Build history of the part. All positions in model axes, mm. A direction names the side the tool comes from. Give positions to 0.01 mm unless a question says otherwise; leave off trailing zeros. Order: outer loops, then holes, each group sorted by start corner. A loop starts at its lowest first (then second) coordinate and runs counter-clockwise, first axis right, second up. Notation, with made-up numbers: (25, 48.25) - (48, 48.25) arc R15 cw to (48, 54.25) - close; hole circle Ø1 at (-9, 4.5). An arc over 180 degrees is marked (long way). Use a Markdown table: item, result.
from build123d import *

# Parameters (mm, degrees)
ESQUISSE1_W             = 80
ESQUISSE1_H             = 80
BOSS_EXTRU_1_DEPTH      = 7
CONG_1_R                = 8
CONG_2_R                = 2
ESQUISSE2_W             = 75
ESQUISSE2_H             = 75
ENL_V_MAT_EXTRU_1_DEPTH = 4
ENL_V_MAT_EXTRU_2_DEPTH = 2
ENL_V_MAT_EXTRU_3_DEPTH = 2
ESQUISSE6_R             = 0.5
ENL_V_MAT_EXTRU_4_DEPTH = 58
CONG_3_R                = 3


with BuildPart() as part:
    # Esquisse1 → Boss.-Extru.1 (new body)
    with BuildSketch(Plane.XY):
        Rectangle(ESQUISSE1_W, ESQUISSE1_H)
    extrude(amount=BOSS_EXTRU_1_DEPTH)

    # Congé1
    cong_1_edges = [part.edges().sort_by_distance(p)[0] for p in [
        (40, -40, 3.5),
        (-40, -40, 3.5),
        (-40, 40, 3.5),
        (40, 40, 3.5),
    ]]
    fillet(cong_1_edges, radius=CONG_1_R)

    # Congé2
    cong_2_edges = [part.edges().sort_by_distance(p)[0] for p in [
        (0, -40, 7),
        (-40, 0, 7),
        (40, 0, 7),
        (0, 40, 7),
        (37.656854249, 37.656854249, 7),
        (37.656854249, -37.656854249, 7),
        (-37.656854249, 37.656854249, 7),
        (-37.656854249, -37.656854249, 7),
    ]]
    fillet(cong_2_edges, radius=CONG_2_R)

    # Esquisse2 → Enlèv. mat.-Extru.1 (cut)
    with BuildSketch(Plane(origin=(0, 0, 0), x_dir=(-1, 0, 0), z_dir=(0, 0, -1))):
        Rectangle(ESQUISSE2_W, ESQUISSE2_H)
    extrude(amount=-ENL_V_MAT_EXTRU_1_DEPTH, mode=Mode.SUBTRACT)

    # Esquisse3 → Enlèv. mat.-Extru.2 (cut)
    with BuildSketch(Plane.XY.offset(7)):
        Polygon((-38, 0), (-23.013072884, 0), (-20.39099813, 2.622074754), (-16.095973356, -8.657779106), (-14.491160811, -12.872434885), (-8.308759443, 7.774506113), (-6.706462268, -5.579927642), (3.046694847, 2.110487656), (8.341678265, 0), (38, 0), (38, 1.552153758), (8.49875294, 1.552153758), (2.797806202, 3.824451283), (-5.535661698, -2.746531659), (-7.678112046, 15.109838358), (-14.491160811, -7.643232416), (-19.53394935, 5.600443877), (-23.634393227, 1.5), (-38, 1.5), align=None)
    extrude(amount=-ENL_V_MAT_EXTRU_2_DEPTH, mode=Mode.SUBTRACT)

    # Esquisse4 → Enlèv. mat.-Extru.3 (cut)
    with BuildSketch(Plane.XY.offset(7)):
        with BuildLine():
            Line((-26.903531704, -27.704969904), (-23.364970672, -31.243530936))
            Line((-23.364970672, -31.243530936), (-19.826409639, -27.704969904))
            ThreePointArc((-19.826409639, -27.704969904), (-20.498887678, -24.324194502), (-23.364970672, -26.239249933))
            ThreePointArc((-23.364970672, -26.239249933), (-26.231053665, -24.324194502), (-26.903531704, -27.704969904))
        make_face()
    extrude(amount=-ENL_V_MAT_EXTRU_3_DEPTH, mode=Mode.SUBTRACT)

    # Esquisse6 → Enlèv. mat.-Extru.4 (cut, through all)
    with BuildSketch(Plane.XY.offset(7)):
        with Locations((11.879182911, 26.878201105)):
            Circle(ESQUISSE6_R)
        with Locations((14.879182911, 26.878201105)):
            Circle(ESQUISSE6_R)
        with Locations((17.879182911, 26.878201105)):
            Circle(ESQUISSE6_R)
        with Locations((20.879182911, 26.878201105)):
            Circle(ESQUISSE6_R)
        with Locations((23.879182911, 26.878201105)):
            Circle(ESQUISSE6_R)
        with Locations((26.879182911, 26.878201105)):
            Circle(ESQUISSE6_R)
        with Locations((29.879182911, 26.878201105)):
            Circle(ESQUISSE6_R)
        with Locations((32.879182911, 26.878201105)):
            Circle(ESQUISSE6_R)
        with Locations((14.879182911, 23.878201105)):
            Circle(ESQUISSE6_R)
        with Locations((17.879182911, 23.878201105)):
            Circle(ESQUISSE6_R)
        with Locations((20.879182911, 23.878201105)):
            Circle(ESQUISSE6_R)
        with Locations((23.879182911, 23.878201105)):
            Circle(ESQUISSE6_R)
        with Locations((26.879182911, 23.878201105)):
            Circle(ESQUISSE6_R)
        with Locations((29.879182911, 23.878201105)):
            Circle(ESQUISSE6_R)
        with Locations((32.879182911, 23.878201105)):
            Circle(ESQUISSE6_R)
        with Locations((14.879182911, 20.878201105)):
            Circle(ESQUISSE6_R)
        with Locations((17.879182911, 20.878201105)):
            Circle(ESQUISSE6_R)
        with Locations((20.879182911, 20.878201105)):
            Circle(ESQUISSE6_R)
        with Locations((23.879182911, 20.878201105)):
            Circle(ESQUISSE6_R)
        with Locations((26.879182911, 20.878201105)):
            Circle(ESQUISSE6_R)
        with Locations((29.879182911, 20.878201105)):
            Circle(ESQUISSE6_R)
        with Locations((32.879182911, 20.878201105)):
            Circle(ESQUISSE6_R)
        with Locations((14.879182911, 17.878201105)):
            Circle(ESQUISSE6_R)
        with Locations((17.879182911, 17.878201105)):
            Circle(ESQUISSE6_R)
        with Locations((20.879182911, 17.878201105)):
            Circle(ESQUISSE6_R)
        with Locations((23.879182911, 17.878201105)):
            Circle(ESQUISSE6_R)
        with Locations((26.879182911, 17.878201105)):
            Circle(ESQUISSE6_R)
        with Locations((29.879182911, 17.878201105)):
            Circle(ESQUISSE6_R)
        with Locations((32.879182911, 17.878201105)):
            Circle(ESQUISSE6_R)
        with Locations((14.879182911, 14.878201105)):
            Circle(ESQUISSE6_R)
        with Locations((17.879182911, 14.878201105)):
            Circle(ESQUISSE6_R)
        with Locations((20.879182911, 14.878201105)):
            Circle(ESQUISSE6_R)
        with Locations((23.879182911, 14.878201105)):
            Circle(ESQUISSE6_R)
        with Locations((26.879182911, 14.878201105)):
            Circle(ESQUISSE6_R)
        with Locations((29.879182911, 14.878201105)):
            Circle(ESQUISSE6_R)
        with Locations((32.879182911, 14.878201105)):
            Circle(ESQUISSE6_R)
        with Locations((11.879182911, 23.878201105)):
            Circle(ESQUISSE6_R)
        with Locations((11.879182911, 20.878201105)):
            Circle(ESQUISSE6_R)
        with Locations((11.879182911, 17.878201105)):
            Circle(ESQUISSE6_R)
        with Locations((11.879182911, 14.878201105)):
            Circle(ESQUISSE6_R)
    enl_v_mat_extru_4 = extrude(amount=-ENL_V_MAT_EXTRU_4_DEPTH, mode=Mode.SUBTRACT)

    # Symétrie2: Enlèv. mat.-Extru.4 across plane
    add(enl_v_mat_extru_4.mirror(Plane.ZX), mode=Mode.SUBTRACT)

    # Congé3
    cong_3_edges = [part.edges().sort_by_distance(p)[0] for p in [
        (-37.5, 37.5, 2),
        (-37.5, -37.5, 2),
        (37.5, -37.5, 2),
        (37.5, 37.5, 2),
    ]]
    fillet(cong_3_edges, radius=CONG_3_R)


solid = part.part
1) Slice it at C-C (y = 9). Write the cut outline in (x, z), and give its area (3 significant figures).
Computed:
| item | result |
|---|---|
| outline | (-40, 0) - (-37.5, 0) - (-37.5, 4) - (37.5, 4) - (37.5, 0) - (40, 0) - (40, 5) arc R2 ccw to (38, 7) - (-6.95, 7) - (-6.95, 5) - (-9.51, 5) - (-9.51, 7) - (-38, 7) arc R2 ccw to (-40, 5) - close |
| area | 253 mm² |
2) Slice it at D-D (z = 6). State how many separate pieces and enclosed holes the cut face has, and give its area (3 significant figures).
Computed:
| item | result |
|---|---|
| separate pieces | 1 |
| enclosed holes | 82 |
| area | 5,980 mm² |
3) Tool access for faces 5 (the flat face through (-21.72, 1.293, 6.014)), 6 (the cylindrical face through (-36.64, -36.6, 2.03)), 7 (the flat face through (0, -40, 2)): list every direction of +Z, -Z, +X, -X, +Y, -Y with a clear straight run to the whole face (end or side of a thin tool).
Computed:
| item | result |
|---|---|
| face 5 | +Z |
| face 6 | -Z |
| face 7 | +Z, -Z, +X, -X, -Y |
4) Slice it at A-A (z = 1.75). Write the cut outline in (x, y).
Computed:
| item | result |
|---|---|
| outline | (-40, -32) arc R8 ccw to (-32, -40) - (32, -40) arc R8 ccw to (40, -32) - (40, 32) arc R8 ccw to (32, 40) - (-32, 40) arc R8 ccw to (-40, 32) - close; hole (-37.5, -34.5) arc R3 ccw to (-34.5, -37.5) - (34.5, -37.5) arc R3 ccw to (37.5, -34.5) - (37.5, 34.5) arc R3 ccw to (34.5, 37.5) - (-34.5, 37.5) arc R3 ccw to (-37.5, 34.5) - close |
5) Two-plate mould, pull along Y, no slides. Class faces 1 (the cylindrical face through (0.45, -39.4, 6.43)), 2 (the flat face through (0, 40, 2)), 3 (the flat face through (-11.443, -2.693, 6.014)), 4 (the flat face through (0, -37.5, 2)): +Y half, -Y half, draft (parallel to the pull), parting line (faces both ways), or undercut.
Computed:
| item | result |
|---|---|
| face 1 | -Y half |
| face 2 | +Y half |
| face 3 | undercut |
| face 4 | undercut |
6) Wall check: line 1 (Y direction, x = -25, z = 1); line 2 (X direction, y = -32.5, z = 0.5); line 3 (X direction, y = 35, z = 0.5). Give the ranges that are in metal, low to high. Write a range as from..to.
Computed:
| item | result |
|---|---|
| line 1 | y = -40..-37.5, 37.5..40 |
| line 2 | x = -39.98..-37.5, 37.5..39.98 |
| line 3 | x = -39.42..-37.46, 37.46..39.42 |
7) Slice it at B-B (x = 0). Write the cut outline in (y, z), and give its area (3 significant figures).
Computed:
| item | result |
|---|---|
| outline | (-40, 0) - (-37.5, 0) - (-37.5, 4) - (37.5, 4) - (37.5, 0) - (40, 0) - (40, 5) arc R2 ccw to (38, 7) - (1.62, 7) - (1.62, 5) - (-0.29, 5) - (-0.29, 7) - (-38, 7) arc R2 ccw to (-40, 5) - close |
| area | 254 mm² |
8) Pin check, flat tips, straight feed: P1, Ø2, axis at x = -34, z = 6, coming from the +Y side; P2, Ø0.8, axis at y = 1, z = 6, coming from the +X side; P3, Ø5, axis at x = -25.44, y = -26.24, coming from the -Z side; P4, Ø1.7, axis at y = 0.5, z = 5.5, coming from the -X side. Stop position of each tip, or through.
Computed:
| item | result |
|---|---|
| P1 | stops at y = 39.87 |
| P2 | stops at x = 39.91 |
| P3 | stops at z = 4 |
| P4 | stops at x = -40 |
